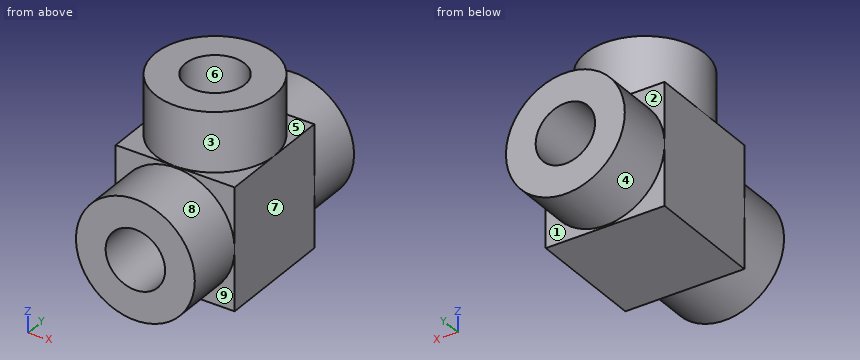
from build123d import *

# Parameters (mm, degrees)
F0_W          = 25.4
F0_H          = 25.4
F1_DEPTH      = 25.9842
F2_R          = 12.7
F2_R_2        = 6.35
F3_DEPTH      = 12.7
F4_R          = 12.7
F4_R_2        = 6.35
F5_DEPTH      = 12.7
F5_DEPTH_BACK = 38.1
F6_R          = 6.35
F7_DEPTH      = 38.101


with BuildPart() as f1:
    # F0 (on Top) → F1 (new body)
    with BuildSketch(Plane.XY):
        Rectangle(F0_W, F0_H)
    extrude(amount=F1_DEPTH)

    # F2 (on face) → F3 (join)
    with BuildSketch(Plane.XY.offset(25.9842)):
        Circle(F2_R)
        Circle(F2_R_2, mode=Mode.SUBTRACT)
    extrude(amount=F3_DEPTH)

    # F4 (on face) → F5 (join, two sides)
    with BuildSketch(Plane.XZ.offset(12.7)) as f5_sk:
        with Locations((0, 12.9921)):
            Circle(F4_R)
        with Locations((0, 12.9921)):
            Circle(F4_R_2, mode=Mode.SUBTRACT)
    extrude(amount=F5_DEPTH)
    extrude(f5_sk.sketch, amount=-F5_DEPTH_BACK)

    # F6 (on face) → F7 (cut, through all)
    with BuildSketch(Plane.XZ.offset(12.7)):
        with Locations((0, 12.9921)):
            Circle(F6_R)
    extrude(amount=-F7_DEPTH, mode=Mode.SUBTRACT)


solid = f1.part
Source: CAD feature listing. Evaluate the final solid. Frame: model axes, mm. Face numbers are marked on the shaded views. A direction names the side the tool comes from. Coordinates: 2 decimals unless noted, no trailing zeros. Loops run counter-clockwise (first coordinate to the right, second up) from the corner with the lowest first, then second, coordinate; pieces in that order, holes last. Notation, with made-up numbers: (47, -32.5) -> (71, -32.5) arc R17 cw to (71, -15.5) -> close; hole circle Ø4 at (82.5, 89.25). An arc over 180 degrees is marked (long way). Answer in a Markdown table with one row per item. Add a question column.
Q1. Section B-B on z = 31. Return the cut outline in (x, y).
Q2. Reachability of the marked faces 1, 2, 3, 4 and 5 from +Z, -Z, +X, -X, +Y, -Y: full face, straight path, thin tool, end or side. Return the list, or none.
Q3. Contact query for flat-ended pins moving along their axis: pin 1 Ø6 at (x, y) = (-5, -19) entering from +Z; pin 2 Ø7.5 at (x, y) = (0, 0) entering from +Z; pin 3 Ø1 at (x, y) = (-6, -17) entering from -Z. Output: stop coordinate, or through.
Q4. Section D-D on z = 14. Return the cut outline in (x, y), and give its area (3 significant figures).
Q5. Section C-C on x = -2.75. Return the cut outline in (y, z), and give its area (3 significant figures).
Q6. Ray query, line 1 along Z through (x, y) = (0, -18.5); line 2 along Y through (x, z) = (0, 30.5); line 3 along Z through (x, y) = (0, -5.25). Return the intervals inside material, ascending.
Q7. Pull-direction query (X, two-part tool) for the marked faces 6, 7, 8 and 9; classes: pulls with the +X half, pulls with the -X half, needs draft (parallel to the pull), parting line crosses it, or undercut.
Q8. Section A-A on y = -2.5. Return the cut outline in (x, z).
Computed values:
| question | item | result |
|---|---|---|
| 1 | outline | circle Ø25.4 at (0, 0); hole circle Ø12.7 at (0, 0) |
| 2 | face 1 | -Z, +Y |
| 2 | face 2 | +Z, +Y |
| 2 | face 3 | +Z |
| 2 | face 4 | +Y |
| 2 | face 5 | +Z, +X, +Y |
| 3 | pin 1 | stops at z = 25.53 |
| 3 | pin 2 | stops at z = 25.98 |
| 3 | pin 3 | stops at z = 1.54 |
| 4 | outline | (-12.7, -12.7) -> (-12.66, -12.7) -> (-12.66, -25.4) -> (-6.27, -25.4) -> (-6.27, 25.4) -> (-12.66, 25.4) -> (-12.66, 12.7) -> (-12.7, 12.7) -> close; (6.27, -25.4) -> (12.66, -25.4) -> (12.66, -12.7) -> (12.7, -12.7) -> (12.7, 12.7) -> (12.66, 12.7) -> (12.66, 25.4) -> (6.27, 25.4) -> close |
| 4 | area | 651 mm^2 |
| 5 | outline | (-25.4, 0.59) -> (-12.7, 0.59) -> (-12.7, 0) -> (12.7, 0) -> (12.7, 0.59) -> (25.4, 0.59) -> (25.4, 7.27) -> (-25.4, 7.27) -> close; (-25.4, 18.72) -> (25.4, 18.72) -> (25.4, 25.39) -> (12.7, 25.39) -> (12.7, 25.98) -> (12.4, 25.98) -> (12.4, 38.68) -> (5.72, 38.68) -> (5.72, 25.98) -> (-5.72, 25.98) -> (-5.72, 38.68) -> (-12.4, 38.68) -> (-12.4, 25.98) -> (-12.7, 25.98) -> (-12.7, 25.39) -> (-25.4, 25.39) -> close |
| 5 | area | 878 mm^2 |
| 6 | line 1 | z = 0.29 to 6.64, 19.34 to 25.69 |
| 6 | line 2 | y = -12.7 to -6.35, 6.35 to 12.7 |
| 6 | line 3 | z = 0 to 6.64, 19.34 to 25.98 |
| 7 | face 6 | undercut |
| 7 | face 7 | pulls with the +X half |
| 7 | face 8 | parting line crosses it |
| 7 | face 9 | needs draft |
| 8 | outline | (-12.7, 0) -> (12.7, 0) -> (12.7, 25.98) -> (12.45, 25.98) -> (12.45, 38.68) -> (5.84, 38.68) -> (5.84, 25.98) -> (-5.84, 25.98) -> (-5.84, 38.68) -> (-12.45, 38.68) -> (-12.45, 25.98) -> (-12.7, 25.98) -> close; hole circle Ø12.7 at (0, 12.99) |
